Geometry check sheet. Reference: the model listing, model coordinates, mm. Give positions to 0.01 mm unless a question says otherwise; leave off trailing zeros. Loops run counter-clockwise (first coordinate to the right, second up) from the corner with the lowest first, then second, coordinate; pieces in that order, holes last. Notation, with made-up numbers: (40, 80.25) - (71, 80.25) arc R21 cw to (71, 101.25) - close; hole circle Ø10 at (-23, -32). An arc over 180 degrees is marked (long way). Use a Markdown table: item, result. Add a question column.
1. Cross-section at B-B on x = 0.5. Enter the section's corners in (y, z).
2. Cross-section at C-C on x = 3. Enter the section's corners in (y, z).
3. Depth check by flat-ended pin: P1, Ø1.3, axis at x = 0, z = -12.45, coming from the -Y side (3 decimals); P2, Ø2, axis at x = -1, z = -13, coming from the -Y side. Enter the tip coordinate at first touch or a pass-through.
4. Cross-section at D-D on z = 14.5. Enter the section's corners in (x, y), and give its area (3 significant figures).
5. Material ranges on L1, parallel to X at y = -1.45, z = -13; L2, parallel to X at y = -0.3, z = -11.5; L3, parallel to Z at x = -2, y = -2.05, recorded low to high.
from build123d import *

# Parameters (mm, degrees)
F0_W     = 10
F0_H     = 34.9
F1_DEPTH = 4
F2_R     = 5
F3_R     = 4.99999
F4_R     = 2.25
F4_R_2   = 1.05
F5_DEPTH = 2
F6_DEPTH = 5


# Not quite as in the source:
# - a fillet or chamfer is up to 0.001 mm smaller than in the source, because OpenCascade refuses the exact size


with BuildPart() as f1:
    # F0 (on Front) → F1 (new body)
    with BuildSketch(Plane.XZ):
        Rectangle(F0_W, F0_H)
    extrude(amount=F1_DEPTH)

    # F2
    f2_edges = [f1.edges().sort_by_distance(p)[0] for p in [
        (5, -2, 17.45),
    ]]
    fillet(f2_edges, radius=F2_R)

    # F3 (radius 5 in the source; OpenCascade refuses exactly that, so slightly less here)
    f3_edges = [f1.edges().sort_by_distance(p)[0] for p in [
        (5, -2, -17.45),
        (-5, -2, -17.45),
    ]]
    fillet(f3_edges, radius=F3_R)

    # F4 (on face) → F5 (cut)
    with BuildSketch(Plane.XZ.offset(4)):
        with Locations((0, -12.45)):
            Circle(F4_R)
        with Locations((0, -12.45)):
            Circle(F4_R_2, mode=Mode.SUBTRACT)
    extrude(amount=-F5_DEPTH, mode=Mode.SUBTRACT)

    # F6 (cut): a face of the model
    f6_faces = [f1.faces().sort_by_distance(p)[0] for p in [
        (0, -4, -12.45),
    ]]
    extrude(f6_faces, amount=-F6_DEPTH, mode=Mode.SUBTRACT)


solid = f1.part
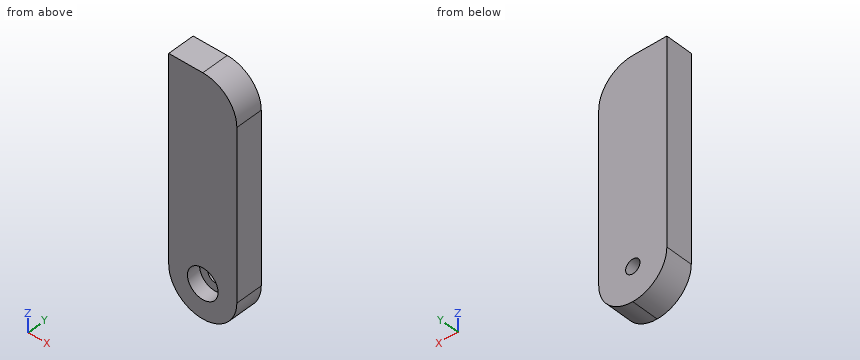
Values found:
| question | item | result |
|---|---|---|
| 1 | outline | (-4, -17.42) - (0, -17.42) - (0, -13.37) - (-2, -13.37) - (-2, -14.64) - (-4, -14.64) - close; (-4, -10.26) - (-2, -10.26) - (-2, -11.53) - (0, -11.53) - (0, 17.42) - (-4, 17.42) - close |
| 2 | outline | (-4, -16.45) - (0, -16.45) - (0, 16.45) - (-4, 16.45) - close |
| 3 | P1 | passes through |
| 3 | P2 | stops at y = -2 |
| 4 | outline | (-5, -4) - (4.56, -4) - (4.56, 0) - (-5, 0) - close |
| 4 | area | 38.2 mm2 |
| 5 | L1 | x = -4.97 to -0.89, 0.89 to 4.97 |
| 5 | L2 | x = -5 to -0.45, 0.45 to 5 |
| 5 | L3 | z = -17.03 to -13.48, -11.42 to 17.45 |
